Geometry: see drawing. Coordinates: mm, zero at the bounding-box minimum. Coordinates: 2 decimals unless noted, no trailing zeros. Write each loop counter-clockwise with the first axis right and the second up, starting at its lowest first coordinate (ties: lowest second). Pieces come first, ordered by that corner, then holes. Notation, with made-up numbers: M 22.5,-18.75 L 34.5,-18.75 A21 cw 34.5,-14.75 Z; hole C -25.75,-40 d3. An arc over 180 degrees is marked long. Write item = value, one per line. Start each with the question number.
1. Section query A-A (x = 75). Output: boundary loops of the cut face in (y, z), then the cut area to 3 significant figures.
2. Line query: line 1 along X through (y, z) = (30, 10); line 2 along Z through (x, y) = (75, 35.5); line 3 along Z through (x, y) = (76, 45.5). Output: solid intervals per line, ascending.
3. Section query B-B (z = 10). Output: boundary loops of the cut face in (x, y), then the cut area to 4 significant figures.
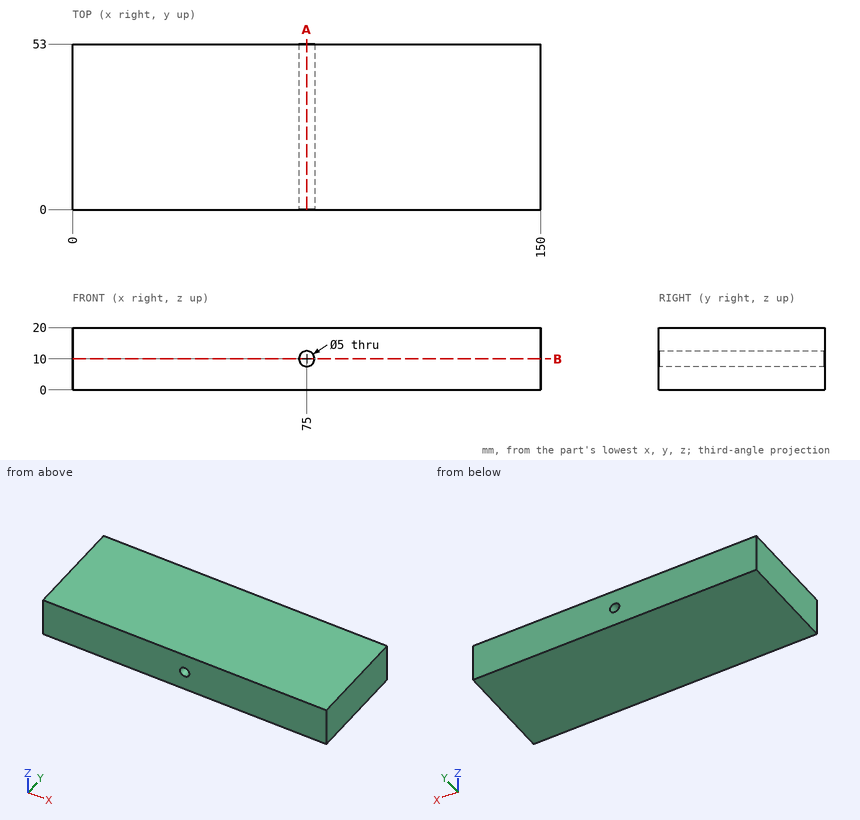
Results are:
q1.outline = M 0,0 L 53,0 L 53,7.5 L 0,7.5 Z; M 0,12.5 L 53,12.5 L 53,20 L 0,20 Z
q1.area = 795 mm^2
q2.line_1 = 0 to 72.5, 77.5 to 150
q2.line_2 = 0 to 7.5, 12.5 to 20
q2.line_3 = 0 to 7.71, 12.29 to 20
q3.outline = M 0,0 L 72.5,0 L 72.5,53 L 0,53 Z; M 77.5,0 L 150,0 L 150,53 L 77.5,53 Z
q3.area = 7,685 mm^2
